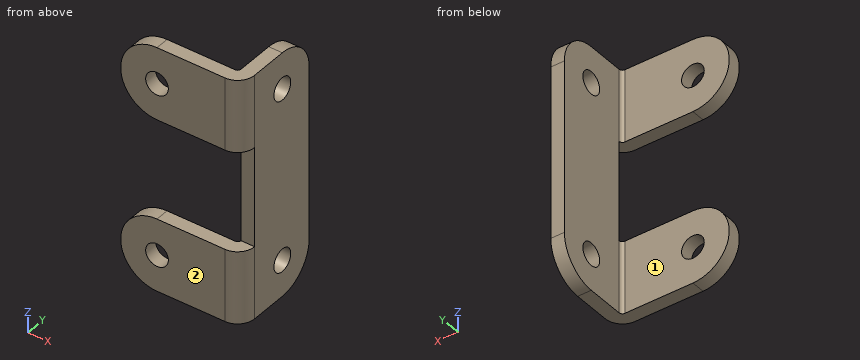
from build123d import *

# Parameters (mm, degrees)
SKETCH1_R          = 2.5
BASE_FLANGE1_DEPTH = 3
EDGE_FLANGE1_DEPTH = 16
SKETCH10_R         = 2.5
CUT_EXTRUDE1_DEPTH = 10
TAB1_START         = -3
TAB1_DEPTH         = 3


# Read off the part's stored shape, not the designer's step: Tab1
# Sheet-metal steps are written as plain solids
with BuildPart() as part:
    # Sketch1 → Base-Flange1 (new body)
    with BuildSketch(Plane(origin=(0, 0, 0), x_dir=(1, 0, 0), z_dir=(0, 1, 0))):
        with BuildLine():
            Line((15, -8), (0, -8))
            ThreePointArc((0, -8), (-8, 0), (0, 8))
            Line((0, 8), (15, 8))
            Line((15, 8), (15, -8))
        make_face()
        with Locations(Location((0, 0, 0), (0, 0, 270))):
            Circle(SKETCH1_R, mode=Mode.SUBTRACT)
    extrude(amount=-BASE_FLANGE1_DEPTH)

    # Edge-Flange1 section (across the edge) → Edge-Flange1 (add)
    with BuildSketch(Plane(origin=(15.7366, 0, 8), x_dir=(-1, 0, 0), z_dir=(0, 0, -1))):
        with BuildLine():
            Line((-3, 0.7366), (-3, 17))
            Line((-3, 17), (0, 17))
            Line((0, 17), (0, 0.7366))
            ThreePointArc((0, 0.7366), (0.215745145, 0.215745145), (0.7366, 0))
            Line((0.7366, 0), (0.7366, -3))
            ThreePointArc((0.7366, -3), (-1.905575199, -1.905575199), (-3, 0.7366))
        make_face()
    extrude(amount=EDGE_FLANGE1_DEPTH)

    # Sketch10 → Cut-Extrude1 (cut)
    with BuildSketch(Plane.ZY.offset(-15.7366)):
        with BuildLine():
            Line((-8, 17), (-8, 9))
            ThreePointArc((-8, 9), (-5.656854249, 14.656854249), (0, 17))
            Line((0, 17), (-8, 17))
        make_face()
        with BuildLine():
            Line((8, 17), (0, 17))
            ThreePointArc((0, 17), (5.656854249, 14.656854249), (8, 9))
            Line((8, 9), (8, 17))
        make_face()
        with Locations(Location((0, 9, 0), (0, 0, 270))):
            Circle(SKETCH10_R)
    extrude(amount=-CUT_EXTRUDE1_DEPTH, mode=Mode.SUBTRACT)


with BuildPart() as body_2:
    # Mirror1: mirrored copy
    add(part.part.mirror(Plane.XY.offset(-19)))


with BuildPart() as part_1:
    add(part.part)

    add(body_2.part)  # Tab1 merges body 2
    # Tab1 outline → Tab1 (add)
    with BuildSketch(Plane.ZY.offset(-15.7366).offset(TAB1_START)):
        with BuildLine():
            ThreePointArc((-8, 9), (-5.656854249, 14.656854249), (0, 17))
            Line((0, 17), (-38, 17))
            ThreePointArc((-38, 17), (-32.343145751, 14.656854249), (-30, 9))
            Line((-30, 9), (-30, 0.7366))
            Line((-30, 0.7366), (-8, 0.7366))
            Line((-8, 0.7366), (-8, 9))
        make_face()
    extrude(amount=TAB1_DEPTH)


solid = part_1.part
Work out the finished part from the listing and answer in its coordinate system (mm). Face numbers are marked on the shaded views. A direction names the side the tool comes from. Coordinates: 2 decimals unless noted, no trailing zeros. Loops run counter-clockwise (first coordinate to the right, second up) from the corner with the lowest first, then second, coordinate; pieces in that order, holes last. Notation, with made-up numbers: (36.25, 39.25) -> (60.25, 39.25) arc R13 cw to (60.25, 52.25) -> close; hole circle Ø10 at (34.5, -11). An arc over 180 degrees is marked (long way). Answer as CSV lines item,"result".
1) The part is cut by section A-A (x = 7.75). Give the vertices of the cut face in (y, z).
A:
outline,"(-3, -46) -> (0, -46) -> (0, -30) -> (-3, -30) -> close; (-3, -8) -> (0, -8) -> (0, 8) -> (-3, 8) -> close"
2) For the marked faces 1 and 2, determine the directions among +Z, -Z, +X, -X, +Y, -Y from which every point of the face is accessible in a straight line to the end or side of a thin tool.
A:
face 1,"+Z, -Z, -X, +Y"
face 2,"+Z, -Z, +X, -X, -Y"
3) Straight lines are drawn through the part: probe 1 along Z at (x, y) = (17.85, 9); probe 2 along Y at (x, z) = (13.5, -4.5); probe 3 along X at (y, z) = (5.25, -11). For each, find the intervals that lie inside material, in ascending order.
A:
probe 1,"z = -46 to -40.5, -35.5 to -2.5, 2.5 to 8"
probe 2,"y = -3 to 0"
probe 3,"x = 15.74 to 18.74"
4) The part is cut by section D-D (z = -23.5). Give the vertices of the cut face in (x, y).
A:
outline,"(15.74, 0.74) -> (18.74, 0.74) -> (18.74, 17) -> (15.74, 17) -> close"
5) Flat-ended cylindrical pins translate along their axes: pin 1 (4 mm diameter, centred on y = 7, z = -30, fed in from -X); pin 2 (3.5 mm diameter, centred on x = 17, z = -18, fed in from -Y); pin 3 (5 mm diameter, centred on x = -1.5, z = -36.5, fed in from +Y). Find the tip coordinate at first contact, or state that the pin passes through.
A:
pin 1,"stops at x = 15.74"
pin 2,"stops at y = 0.74"
pin 3,"stops at y = 0"
6) The part is cut by section C-C (y = 10). Give the vertices of the cut face in (x, z), and give its area (3 significant figures).
A:
outline,"(15.74, -45.94) -> (18.74, -45.94) -> (18.74, -40.29) -> (15.74, -40.29) -> close; (15.74, -35.71) -> (18.74, -35.71) -> (18.74, -2.29) -> (15.74, -2.29) -> close; (15.74, 2.29) -> (18.74, 2.29) -> (18.74, 7.94) -> (15.74, 7.94) -> close"
area,"134 mm²"
7) The part is cut by section B-B (x = 17). Give the vertices of the cut face in (y, z).
A:
outline,"(-2.42, -46) -> (9, -46) arc R8 ccw to (17, -38) -> (17, 0) arc R8 ccw to (9, 8) -> (-2.42, 8) -> (-2.42, -8) -> (0.74, -8) -> (0.74, -30) -> (-2.42, -30) -> close; hole circle Ø5 at (9, -38); hole circle Ø5 at (9, 0)"
